Solid Edge part; units mm, degrees
sketch "Sketch1" plane through (0, 0, 0) normal (0, -1, 0) x (1, 0, 0)
  line L0 (-37.5, -55) -> (37.5, -55)
  line L1 (37.5, -55) -> (37.5, 55)
  line L2 (37.5, 55) -> (-37.5, 55)
  line L3 (-37.5, 55) -> (-37.5, -55)
  line L4 (-42.5, -60) -> (42.5, -60)
  line L5 (42.5, -60) -> (42.5, 60)
  line L6 (42.5, 60) -> (-42.5, 60)
  line L7 (-42.5, 60) -> (-42.5, -60)
extrude "Protrusion1" add sketch "Sketch1" along normal blind 60
sketch "Sketch2" plane through (0, -60, 0) normal (0, -1, 0) x (1, 0, 0)
  circle A0 centre (30, -25) radius 10
  circle A1 centre (-30, -25) radius 10
  dimension "D1" = 30
  dimension "D2" = 30
extrude "camera_cut" cut sketch "Sketch2" against normal blind 20
sketch "Sketch3" plane through (0, -56, 0) normal (0, -1, 0) x (1, 0, 0)
  line L0 (-33, -55) -> (-25, -55)
  line L1 (-25, -55) -> (-25, -52)
  arc A0 (-33, -52) -> (-25, -52) centre (-29, -52) cw
  line L2 (-33, -55) -> (-33, -52)
  circle A1 centre (0, 52) radius 1.25
  circle A2 centre (-29, -52) radius 1.25
  line L3 (25, -55) -> (33, -55)
  line L4 (33, -55) -> (33, -52)
  arc A3 (25, -52) -> (33, -52) centre (29, -52) cw
  line L5 (25, -55) -> (25, -52)
  circle A4 centre (29, -52) radius 1.25
  arc A5 (-4, 52) -> (4, 52) centre (0, 52) ccw
  line L6 (4, 55) -> (4, 52)
  line L7 (-4, 55) -> (4, 55)
  line L8 (-4, 55) -> (-4, 52)
  dimension "D1" = 4
  dimension "D2" = 4
  dimension "D3" = 25
extrude "mounting_bottom" add sketch "Sketch3" against normal blind 5
properties material "Nylon, allgemein"
The listing builds one solid part. Answer for the finished solid, in the listing's coordinates (mm). A direction names the side the tool comes from. Give positions to 0.01 mm unless a question says otherwise; leave off trailing zeros. Loops run counter-clockwise (first coordinate to the right, second up) from the corner with the lowest first, then second, coordinate; pieces in that order, holes last. Notation, with made-up numbers: M 54.5,84.5 L 102.5,84.5 A11 cw 102.5,96.5 Z; hole C 42.25,33.5 d5. An arc over 180 degrees is marked long. Answer as CSV lines item,"result".
Item 1: Given pin 1 Ø3 at (x, z) = (0, 52) entering from +Y; pin 2 Ø1.2 at (x, z) = (-39, -22.5) entering from -Y; pin 3 Ø3.5 at (x, z) = (27.5, -52) entering from -Y, each flat-ended and moving along its own axis, determine where each tip first touches the part or whether it passes through.
Values follow:
pin 1,"stops at y = -51"
pin 2,"stops at y = -40"
pin 3,"stops at y = -56"
Item 2: The part is cut by section A-A (x = 15.5). Give the vertices of the cut face in (y, z), and give its area (3 significant figures).
Values follow:
outline,"M -60,-60 L 0,-60 L 0,-55 L -60,-55 Z; M -60,55 L 0,55 L 0,60 L -60,60 Z"
area,"600 mm^2"
Item 3: Straight lines are drawn through the part: line 1 along Z through (x, y) = (0, -52.35); line 2 along X through (y, z) = (-27.5, -42); line 3 along Z through (x, y) = (6, -51). For each, find the intervals that lie inside material, in ascending order. Write a range as [from, to].
Values follow:
line 1,"z = [-60, -55], [48, 50.75], [53.25, 60]"
line 2,"x = [-42.5, -37.5], [37.5, 42.5]"
line 3,"z = [-60, -55], [55, 60]"
Item 4: The part is cut by section B-B (y = -44). Give the vertices of the cut face in (x, z), and give its area (3 significant figures).
Values follow:
outline,"M -42.5,-60 L 42.5,-60 L 42.5,60 L -42.5,60 Z; hole M -37.5,-55 L 37.5,-55 L 37.5,-31.61 A10 ccw 37.5,-18.39 L 37.5,55 L -37.5,55 L -37.5,-18.39 A10 ccw -37.5,-31.61 Z"
area,"1,900 mm^2"
Item 5: Which of the six approach directions +Z, -Z, +X, -X, +Y, -Y give full straight-line access (tool end or side, diameter ignored) to faces 3 (the flat face through (28, -56, -51)), 4 (the flat face through (-1, -51, 51)), 5 (the flat face through (-37.5, -30, 1))?
Values follow:
face 3,"-Y"
face 4,"+Y"
face 5,"+Y, -Y"
Item 6: The part is cut by section D-D (y = -53). Give the vertices of the cut face in (x, z), and give its area (3 significant figures).
Values follow:
outline,"M -42.5,-60 L 42.5,-60 L 42.5,60 L -42.5,60 Z; hole M -37.5,-55 L -33,-55 L -33,-52 A4 cw -25,-52 L -25,-55 L 25,-55 L 25,-52 A4 cw 33,-52 L 33,-55 L 37.5,-55 L 37.5,-31.61 A10 ccw 37.5,-18.39 L 37.5,55 L 4,55 L 4,52 A4 cw -4,52 L -4,55 L -37.5,55 L -37.5,-18.39 A10 ccw -37.5,-31.61 Z; hole C -29,-52 d2.5; hole C 0,52 d2.5; hole C 29,-52 d2.5"
area,"2,040 mm^2"
Item 7: The mould has two halves that part along X. Classify faces 1 (the cylindrical face through (0, -54, 48)), 2 (the flat face through (1, -30, 60)): released by +X, released by -X, zero draft, split by the parting line, or undercut.
Values follow:
face 1,"undercut"
face 2,"zero draft"
Item 8: The part is cut by section C-C (z = 26.5). Give the vertices of the cut face in (x, y), and give its area (3 significant figures).
Values follow:
outline,"M -42.5,-60 L -37.5,-60 L -37.5,0 L -42.5,0 Z; M 37.5,-60 L 42.5,-60 L 42.5,0 L 37.5,0 Z"
area,"600 mm^2"
